The listing builds one solid part. Answer for the finished solid, in the listing's coordinates (mm). A direction names the side the tool comes from. Give positions to 0.01 mm unless a question says otherwise; leave off trailing zeros. Loops run counter-clockwise (first coordinate to the right, second up) from the corner with the lowest first, then second, coordinate; pieces in that order, holes last.
Item 1: A tool of negligible diameter and unlimited length cuts with its end or side. For faces 4 (the face through (26.75, -19, 16)), 5 (the face through (-13.699, -8.285, 13.479)), 6 (the face through (4, -6, 13)), from which of +Z, -Z, +X, -X, +Y, -Y can it reach the whole face along a straight path? Write none if from no direction.
Item 2: The mould has two halves that part along X. Classify faces 1 (the face through (-19, -31, 13)), 2 (the face through (-19.248, -35.287, 14.282)), 3 (the face through (26.037, -33.998, 15.74)): pulls with the +X half, pulls with the -X half, needs draft (parallel to the pull), parting line crosses it, or undercut.
Item 3: Each of these flat-tipped pins is pushed along its axis until it touches: pin 1 Ø15.5 at (x, y) = (8, -21) entering from -Z; pin 2 Ø1 at (x, z) = (-19, 12.5) entering from +Y; pin 3 Ø1.4 at (x, z) = (26.5, 12.5) entering from +Y; pin 4 Ø10 at (x, y) = (2, -9.5) entering from +Z. Where does it stop, or does it pass through?
Item 4: Section A-A, the plane x = 12 is taken. Give the vertices of the cut face in (y, z).
Item 5: Section B-B, the plane z = 12.6 is taken. Give the vertices of the cut face in (x, y), and give its area (3 significant figures).
Item 6: Section D-D, the plane y = -12.5 is taken. Give the vertices of the cut face in (x, z), and give its area (4 significant figures).
Item 7: Section C-C, the plane y = -23 is taken. Give the vertices of the cut face in (x, z), and give its area (3 significant figures).
Item 8: Consider line 1 along Y through (x, z) = (14.5, 14.1); line 2 along X through (y, z) = (-25, 15.95); line 3 along Y through (x, z) = (-9.5, 13.4). Determine where each line is inside the solid, lowest interval first.
from build123d import *

# Parameters (mm, degrees)
SKETCH135_W             = 30
SKETCH135_H             = 48
PAD050_DEPTH            = 4.5
SKETCH137_W             = 3
SKETCH137_H             = 39
SKETCH137_W_2           = 21
SKETCH137_H_2           = 44
POCKET047_DEPTH         = 5
FILLET058_R             = 3
FILLET059_R             = 2.5
FILLET060_R             = 1
SKETCH138_W             = 30
SKETCH138_H             = 45.5
POCKET048_DEPTH         = 1.5
FILLET061_R             = 2.5
SKETCH139_W             = 20
SKETCH139_H             = 4
POCKET049_DEPTH         = 48.001
FILLET062_R             = 0.5
BODY057_PLACEMENT_ANGLE = 90


with BuildPart() as part:
    # Sketch135 → Pad050 (new body)
    with BuildSketch(Plane.XY):
        Rectangle(SKETCH135_W, SKETCH135_H)
    extrude(amount=PAD050_DEPTH)

    # Sketch137 (on Face6 of Pad050) → Pocket047 (cut)
    with BuildSketch(Plane.XY.offset(4.5)):
        with Locations((11.5, -1.5)):
            Rectangle(SKETCH137_W, SKETCH137_H)
        with Locations((-2.5, 0)):
            Rectangle(SKETCH137_W_2, SKETCH137_H_2)
    extrude(amount=-POCKET047_DEPTH, mode=Mode.SUBTRACT)

    # Fillet058
    fillet058_edges = [part.edges().sort_by_distance(p)[0] for p in [
        (8, 22, 2.25),
        (-13, 22, 2.25),
        (8, -22, 2.25),
        (-13, -22, 2.25),
    ]]
    fillet(fillet058_edges, radius=FILLET058_R)

    # Fillet059
    fillet059_edges = [part.edges().sort_by_distance(p)[0] for p in [
        (-15, 24, 2.25),
        (-15, -24, 2.25),
        (15, 24, 2.25),
        (15, -24, 2.25),
    ]]
    fillet(fillet059_edges, radius=FILLET059_R)

    # Fillet060
    fillet060_edges = [part.edges().sort_by_distance(p)[0] for p in [
        (10, 18, 2.25),
        (13, 18, 2.25),
        (13, -21, 2.25),
        (10, -21, 2.25),
    ]]
    fillet(fillet060_edges, radius=FILLET060_R)

    # Sketch138 (on Face26 of Fillet060) → Pocket048 (cut)
    with BuildSketch(Plane.XY.offset(4.5)):
        with Locations((1.25, 0)):
            Rectangle(SKETCH138_W, SKETCH138_H)
    extrude(amount=-POCKET048_DEPTH, mode=Mode.SUBTRACT)

    # Fillet061
    fillet061_edges = [part.edges().sort_by_distance(p)[0] for p in [
        (-13.75, 22.75, 3.75),
        (-13.75, -22.75, 3.75),
    ]]
    fillet(fillet061_edges, radius=FILLET061_R)

    # Sketch139 (on Face27 of Fillet061) → Pocket049 (cut, through all)
    with BuildSketch(Plane.XZ.offset(24)):
        with Locations((0, -0.25)):
            Rectangle(SKETCH139_W, SKETCH139_H)
    extrude(amount=-POCKET049_DEPTH, mode=Mode.SUBTRACT)

    # Fillet062
    fillet062_edges = [part.edges().sort_by_distance(p)[0] for p in [
        (-10, -23, 1.75),
        (-10, 23, 1.75),
    ]]
    fillet(fillet062_edges, radius=FILLET062_R)


with BuildPart() as part_1:
    # Body057 placement: moved
    add(part.part.moved(Location((4, -21, 12))).rotate(Axis((4, -21, 12), (0, 0, 1)), BODY057_PLACEMENT_ANGLE))


solid = part_1.part
Worked answers:
1. face 4: +Z, +Y
1. face 5: +Z, -Z
1. face 6: +Z, -Z, +X, -X, +Y
2. face 1: needs draft
2. face 2: pulls with the -X half
2. face 3: undercut
3. pin 1: passes through
3. pin 2: stops at y = -6.21
3. pin 3: stops at y = -6.02
3. pin 4: stops at z = 15
4. outline: (-36, 12) - (-34, 12) - (-34, 15) - (-34.75, 15) - (-34.75, 16.5) - (-36, 16.5) - close; (-13, 13.75) - (-11, 13.75) - (-11, 15) - (-13, 15) - close; (-8, 12) - (-6, 12) - (-6, 15) - (-8, 15) - close
5. outline: (-20, -33.5) arc R2.5 ccw to (-17.5, -36) - (25.5, -36) arc R2.5 ccw to (28, -33.5) - (28, -31) - (26, -31) arc R3 cw to (23, -34) - (-15, -34) arc R3 cw to (-18, -31) - (-20, -31) - close; (-20, -11) - (-13, -11) arc R1 cw to (-14, -10) - (-14, -9) arc R1 cw to (-13, -8) - (24, -8) arc R1 cw to (25, -9) - (25, -10) arc R1 cw to (24, -11) - (28, -11) - (28, -8.5) arc R2.5 ccw to (25.5, -6) - (-17.5, -6) arc R2.5 ccw to (-20, -8.5) - close
5. area: 230 mm2
6. outline: (-20, 13.75) - (28, 13.75) - (28, 16.5) - (26.75, 16.5) - (26.75, 15) - (-18.75, 15) - (-18.75, 16.5) - (-20, 16.5) - close
6. area: 63.75 mm2
7. outline: (-20, 13.75) - (-18, 13.75) - (-18, 15) - (-18.75, 15) - (-18.75, 16.5) - (-20, 16.5) - close; (26, 13.75) - (28, 13.75) - (28, 16.5) - (26.75, 16.5) - (26.75, 15) - (26, 15) - close
7. area: 8.75 mm2
8. line 1: y = -36 to -34, -13 to -11, -8 to -6
8. line 2: x = -20 to -18.75, 26.75 to 28
8. line 3: y = -36 to -34, -8 to -6
